from build123d import *

# Parameters (mm, degrees)
F0_R            = 11
F1_DEPTH        = 4.2
F3_DEPTH        = 4.201
F3_COPIES_COUNT = 12
F5_R            = 3.2
F6_DEPTH        = 3
F7_W            = 3.4390550572
F7_H            = 3.9651677944
F8_DEPTH        = 7.201


# Not quite as in the source:
# - a pattern or mirror of a feature is missing from the dataset's text; its kind, count and spacing are read off the source's solid


with BuildPart() as f1:
    # F0 (on Top) → F1 (new body)
    with BuildSketch(Plane.XY):
        Circle(F0_R)
    extrude(amount=F1_DEPTH)

    # F2 (on face) → F3 (cut, through all)
    with BuildSketch(Plane(origin=(0, 0, 0), x_dir=(1, 0, 0), z_dir=(0, 0, -1))):
        with BuildLine():
            Line((-10.5683914605, 3.0510820928), (-6.7253400203, 1.9415976954))
            ThreePointArc((-6.7253400203, 1.9415976954), (-6.6904301664, 2.0586753481), (-6.6534823425, 2.1751259084))
            Line((-6.6534823425, 2.1751259084), (-9.6111801384, 5.3502538582))
            ThreePointArc((-9.6111801384, 5.3502538582), (-10.1550640166, 4.2278451744), (-10.5683914605, 3.0510820928))
        make_face()
        with BuildLine():
            ThreePointArc((-6.7890039073, 1.7057039447), (-6.7582012706, 1.8239286132), (-6.7253400203, 1.9415976954))
            Line((-6.7253400203, 1.9415976954), (-10.5683914605, 3.0510820928))
            ThreePointArc((-10.5683914605, 3.0510820928), (-10.8458486133, 1.8350934191), (-10.9838684057, 0.5955122546))
            Line((-10.9838684057, 0.5955122546), (-6.7890039073, 1.7057039447))
        make_face()
    f3 = extrude(amount=-F3_DEPTH, mode=Mode.SUBTRACT)

    # F3_copies: F3 ×12 about axis
    f3_copies_axis = Axis((0, 0, 0), (0, 0, 1))
    for i in range(1, F3_COPIES_COUNT):
        add(f3.rotate(f3_copies_axis, i * 360 / F3_COPIES_COUNT), mode=Mode.SUBTRACT)

    # F5 (on face) → F6 (join)
    with BuildSketch(Plane.XY.offset(4.2)):
        Circle(F5_R)
    extrude(amount=F6_DEPTH)

    # F7 (on face) → F8 (cut, through all)
    with BuildSketch(Plane.XY.offset(7.2)):
        Rectangle(F7_W, F7_H)
    extrude(amount=-F8_DEPTH, mode=Mode.SUBTRACT)


solid = f1.part
Could you check a few things on this model? Use its own coordinates, in mm. A direction names the side the tool comes from. Give positions to 0.01 mm unless a question says otherwise; leave off trailing zeros. Write each loop counter-clockwise with the first axis right and the second up, starting at its lowest first coordinate (ties: lowest second). Pieces come first, ordered by that corner, then holes. Notation, with made-up numbers: (34, 4.5) -> (91, 4.5) arc R18 cw to (91, 14.5) -> close; hole circle Ø11 at (29, -32.5). An arc over 180 degrees is marked (long way). Write each question's results on one line, items separated by ' | '. Start each with the question number.
Q1. Suppose I cut it at B-B, the plane x = -7.5. List the corners of the cut face in (y, z) for me.
Q2. I'm going to push flat-ended pins straight in: pin 1 Ø5 at (x, y) = (7.5, -8.5) entering from +Z; pin 2 Ø1.5 at (y, z) = (0, 6) entering from -X; pin 3 Ø4 at (x, z) = (0, 4.5) entering from -Y; pin 4 Ø3 at (y, z) = (-4.5, 3.5) entering from +X. Where does each tip first touch, or does it pass through?
Q3. I need wall thicknesses on probe 1 along X at (y, z) = (-9.5, 2.5); probe 2 along Y at (x, z) = (-9.25, 2); probe 3 along Z at (x, y) = (-0.25, -4.25). Which ranges of each line are inside material? Lowest first, please.
Q4. Suppose I cut it at A-A, the plane z = 5.25. List the corners of the cut face in (x, y) for me, and give its area (3 significant figures).
Q5. Suppose I cut it at C-C, the plane x = -3.5. List the corners of the cut face in (y, z) for me.
Q6. Which directions (+Z, -Z, +X, -X, +Y, -Y) give clear straight access to the entire face, cutting with the end or side of a thin tool? Please do faces 1 (the face through (1.72, 0, 4)), 2 (the face through (-8.11, -3.74, 2.07)), 3 (the face through (0.816, 8.895, 2.071)).
Outcome:
1) outline: (-5.54, 0) -> (-3.08, 0) -> (-3.08, 4.2) -> (-5.54, 4.2) -> close; (-1.52, 0) -> (1.24, 0) -> (1.24, 4.2) -> (-1.52, 4.2) -> close; (2.68, 0) -> (5.2, 0) -> (5.2, 4.2) -> (2.68, 4.2) -> close
2) pin 1: z = 4.2 | pin 2: x = -3.2 | pin 3: y = -11 | pin 4: x = 9.81
3) probe 1: -5.55 to -4.67, -0.63 to 0.99, 5.23 to 5.55 | probe 2: -5.95 to -4.96, -1.05 to 0.71, 4.42 to 5.6 | probe 3: 0 to 4.2
4) outline: circle Ø6.4 at (0, 0); hole (-1.72, -1.98) -> (1.72, -1.98) -> (1.72, 1.98) -> (-1.72, 1.98) -> close | area: 18.5 mm2
5) outline: (-8.32, 0) -> (7.89, 0) -> (7.89, 4.2) -> (-8.32, 4.2) -> close
6) face 1: +Z, -Z | face 2: +Z, -Z, -X | face 3: +Z, -Z, +Y
